Source: CAD feature listing. Evaluate the final solid. Frame: model axes, mm. Face numbers are marked on the shaded views. A direction names the side the tool comes from. Round coordinates to 2 decimals unless told otherwise and drop trailing zeros. Write each loop counter-clockwise with the first axis right and the second up, starting at its lowest first coordinate (ties: lowest second). Pieces come first, ordered by that corner, then holes. Notation, with made-up numbers: M 5.5,75.25 L 9.5,75.25 A28 ccw 9.5,103.25 Z; hole C -17.5,-22.5 d3. An arc over 180 degrees is marked long. Answer in a Markdown table with one row per item. Add a question column.
Item 1: Mould query, pull axis X, two halves, no side actions, for the marked faces 4, 5, 6 and 7. Classes: released by +X, released by -X, zero draft, split by the parting line, or undercut.
Item 2: Set-up query: the marked faces 1, 2 and 3. Return all of +Z, -Z, +X, -X, +Y, -Y with unobstructed straight access to the full face (end or side cutting, diameter ignored); none if empty.
Item 3: Cut plane A-A on y = 5. Return loops of the section in (x, z) (1 decimal).
Item 4: Contact query for flat-ended pins moving along their axis: pin 1 (10 mm diameter, centred on x = -4.5, y = 7.5, fed in from -Z); pin 2 (6.5 mm diameter, centred on y = 12, z = 2, fed in from -X); pin 3 (5 mm diameter, centred on x = 4.5, y = 4, fed in from -Z); pin 4 (8 mm diameter, centred on y = 3, z = 1, fed in from +X). Output: stop coordinate, or through.
Item 5: Material intervals for probe 1 along X at (y, z) = (14, 1); probe 2 along Y at (x, z) = (9.5, -0.25); probe 3 along X at (y, z) = (11.25, 0), sorted ascending.
Item 6: Cut plane C-C on y = 7.75. Return loops of the section in (x, z) (1 decimal).
Item 7: Cut plane B-B on z = 1.25. Return loops of the section in (x, y).
Item 8: Cut plane D-D on y = 14.75. Return loops of the section in (x, z).
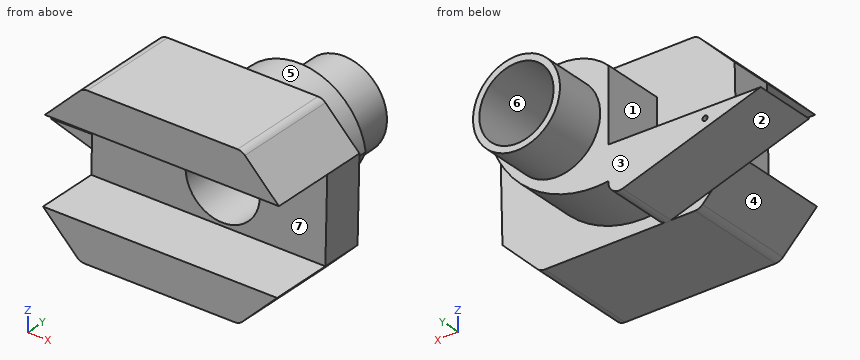
from build123d import *

# Parameters (mm, degrees)
BOSS_EXTRUDE2_DEPTH = 10
CUT_EXTRUDE2_DEPTH  = 6
BOSS_EXTRUDE4_DEPTH = 6
SKETCH6_R           = 4.1
BOSS_EXTRUDE5_DEPTH = 5
SKETCH8_R           = 3.5
CUT_EXTRUDE3_DEPTH  = 15
SKETCH9_R           = 0.238796938
CUT_EXTRUDE4_DEPTH  = 5
FILLET3_R           = 1
FILLET5_R           = 1


with BuildPart() as part:
    # Sketch1 → Boss-Extrude2 (new body)
    with BuildSketch(Plane(origin=(0, 0, 0), x_dir=(1, 0, 0), z_dir=(0, 1, 0))):
        Polygon((8.212445626, 7.40100076), (-6.787554374, 7.224195263), (-10.281169213, 3.647233513), (-10.104363716, -4.352766487), (-6.527401966, -7.846381326), (8.472598034, -7.669575828), (11.966212872, -4.092614079), (11.789407375, 3.907385921), align=None)
    extrude(amount=BOSS_EXTRUDE2_DEPTH)

    # Sketch4 → Cut-Extrude2 (cut)
    with BuildSketch(Plane(origin=(0, 0, 0), x_dir=(1, 0, 0), z_dir=(0, 1, 0))):
        Polygon((-10.281169213, 3.647233513), (11.789407375, 3.907385921), (11.966212872, -4.092614079), (-10.104363716, -4.352766487), align=None)
    extrude(amount=CUT_EXTRUDE2_DEPTH, mode=Mode.SUBTRACT)

    # Sketch5 → Boss-Extrude4 (add)
    with BuildSketch(Plane(origin=(0, 10, 0), x_dir=(1, 0, 0), z_dir=(0, 1, 0))):
        with BuildLine():
            Line((-17.121590923, 2.980762336), (-4.095095114, 7.255931369))
            ThreePointArc((-4.095095114, 7.255931369), (-3.125179525, 7.071252821), (-2.766206415, 6.151480718))
            ThreePointArc((-2.766206415, 6.151480718), (3.686890427, 4.860901674), (8.008746735, -0.10192123))
            ThreePointArc((8.008746735, -0.10192123), (3.769808673, -5.271440115), (-2.766206415, -3.866794904))
            Line((-2.766206415, -3.866794904), (-2.766206415, 2.980762336))
            Line((-2.766206415, 2.980762336), (-17.121590923, 2.980762336))
        make_face()
    extrude(amount=BOSS_EXTRUDE4_DEPTH)

    # Sketch6 → Boss-Extrude5 (add)
    with BuildSketch(Plane(origin=(0, 16, 0), x_dir=(1, 0, 0), z_dir=(0, 1, 0))):
        with Locations((2.116284808, 0)):
            Circle(SKETCH6_R)
    extrude(amount=BOSS_EXTRUDE5_DEPTH)

    # Sketch8 → Cut-Extrude3 (cut)
    with BuildSketch(Plane(origin=(0, 21, 0), x_dir=(1, 0, 0), z_dir=(0, 1, 0))):
        with Locations((2.116284808, 0)):
            Circle(SKETCH8_R)
    extrude(amount=-CUT_EXTRUDE3_DEPTH, mode=Mode.SUBTRACT)

    # Sketch9 → Cut-Extrude4 (cut)
    with BuildSketch(Plane(origin=(0, 16, 0), x_dir=(1, 0, 0), z_dir=(0, 1, 0))):
        with Locations((-11.868205528, 3.862890266)):
            Circle(SKETCH9_R)
    extrude(amount=-CUT_EXTRUDE4_DEPTH, mode=Mode.SUBTRACT)

    # Fillet3
    fillet3_edges = [part.edges().sort_by_distance(p)[0] for p in [
        (8.472598034, 5, 7.669575828),
    ]]
    fillet(fillet3_edges, radius=FILLET3_R)

    # Fillet5
    fillet5_edges = [part.edges().sort_by_distance(p)[0] for p in [
        (-6.527401966, 5, 7.846381326),
        (-6.787554374, 5, -7.224195263),
        (8.212445626, 5, -7.40100076),
    ]]
    fillet(fillet5_edges, radius=FILLET5_R)


solid = part.part
Results below:
| question | item | result |
|---|---|---|
| 1 | face 4 | released by -X |
| 1 | face 5 | split by the parting line |
| 1 | face 6 | undercut |
| 1 | face 7 | zero draft |
| 2 | face 1 | +Z, -X, +Y |
| 2 | face 2 | -Z, -X, +Y |
| 2 | face 3 | +Y |
| 3 | outline | M -10.3,-3.6 L -7.1,-6.9 A1 ccw -6.4,-7.2 L 7.8,-7.4 A1 ccw 8.5,-7.1 L 11.8,-3.9 Z; M -10.1,4.4 L 12,4.1 L 8.8,7.4 A1 ccw 8.1,7.7 L -6.1,7.8 A1 ccw -6.8,7.6 Z |
| 4 | pin 1 | z = -7.31 |
| 4 | pin 2 | x = -10.21 |
| 4 | pin 3 | z = -7.39 |
| 4 | pin 4 | x = 11.97 |
| 5 | probe 1 | -2.77 to -1.24, 5.47 to 7.82 |
| 5 | probe 2 | 6 to 10 |
| 5 | probe 3 | -2.77 to -1.38, 5.62 to 7.97 |
| 6 | outline | M -10.3,-3.6 L -7.1,-6.9 A1 ccw -6.4,-7.2 L 7.8,-7.4 A1 ccw 8.5,-7.1 L 11.8,-3.9 L 12,4.1 L 8.8,7.4 A1 ccw 8.1,7.7 L -6.1,7.8 A1 ccw -6.8,7.6 L -10.1,4.4 Z; hole C 2.1,0 d7 |
| 7 | outline | M -10.17,6 L -1.15,6 L -1.15,21 L -1.79,21 L -1.79,16 L -2.77,16 L -2.77,10 L -10.17,10 Z; M 5.39,6 L 11.9,6 L 11.9,10 L 7.74,10 L 7.74,16 L 6.02,16 L 6.02,21 L 5.39,21 Z |
| 8 | outline | M -17.12,-2.98 L -4.1,-7.26 A1.02 ccw -2.77,-6.15 A10.2 ccw 8.01,0.1 A6.42 ccw -2.77,3.87 L -2.77,-2.98 Z; hole C -11.87,-3.86 d0.48; hole C 2.12,0 d7 |
